Work out the finished part from the listing and answer in its coordinate system (mm). Face numbers are marked on the shaded views. Round coordinates to 2 decimals unless told otherwise and drop trailing zeros. Write each loop counter-clockwise with the first axis right and the second up, starting at its lowest first coordinate (ties: lowest second). Pieces come first, ordered by that corner, then holes. Notation, with made-up numbers: (12.25, 16.25) - (69.25, 16.25) arc R16 ccw to (69.25, 40.25) - close; hole circle Ø8 at (1.25, -20.5). An arc over 180 degrees is marked (long way). Answer as a JSON object with one key per item and string values.
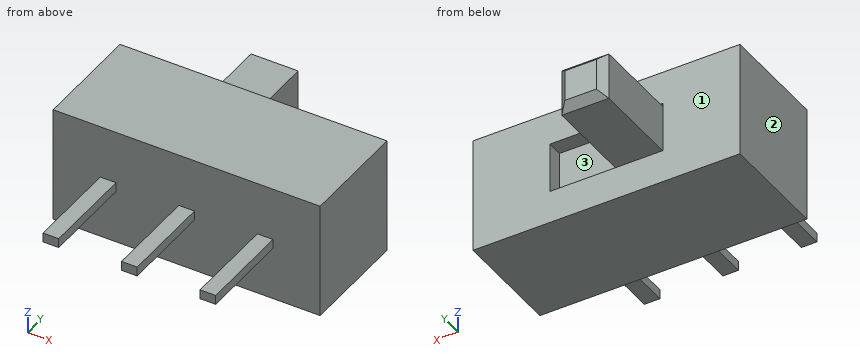
Autodesk Inventor part; units mm, degrees
ref_plane "YZ Plane" through (0, 0, 0) normal (1, 0, 0) x (0, 1, 0)
ref_plane "XZ Plane" through (0, 0, 0) normal (0, 1, 0) x (-1, 0, 0)
ref_plane "XY Plane" through (0, 0, 0) normal (0, 0, 1) x (1, 0, 0)
sketch "Sketch1" plane through (0, 0, 0) normal (0, 1, 0) x (-1, 0, 0)
  line L0 (4.25, -1.85) -> (-4.25, -1.85)
  line L1 (-4.25, -1.85) -> (-4.25, 1.85)
  line L2 (-4.25, 1.85) -> (4.25, 1.85)
  line L3 (4.25, 1.85) -> (4.25, -1.85)
  point P0 (0, 0)
  point P1 (4.25, 0)
  point P2 (0, -1.85)
  dimension "d0" = 8.5
  dimension "d1" = 3.7
extrude "Extrusion1" add sketch "Sketch1" along normal blind 3.5
sketch "Sketch2" plane through (0, 0, 0) normal (0, -1, 0) x (1, 0, 0)
  line L0 (4.25, 1.85) -> (-4.25, 1.85)
  line L1 (-2.75, 0.15) -> (-2.25, 0.15)
  line L2 (-2.25, 0.15) -> (-2.25, -0.15)
  line L3 (-2.25, -0.15) -> (-2.75, -0.15)
  line L4 (-2.75, -0.15) -> (-2.75, 0.15)
  line L5 (-0.25, 0.15) -> (0.25, 0.15)
  line L6 (0.25, 0.15) -> (0.25, -0.15)
  line L7 (0.25, -0.15) -> (-0.25, -0.15)
  line L8 (-0.25, -0.15) -> (-0.25, 0.15)
  line L9 (2.25, 0.15) -> (2.75, 0.15)
  line L10 (2.75, 0.15) -> (2.75, -0.15)
  line L11 (2.75, -0.15) -> (2.25, -0.15)
  line L12 (2.25, -0.15) -> (2.25, 0.15)
  point P0 (0, 0)
  point P1 (-2.75, 0)
  point P2 (-2.5, 0.15)
  point P3 (-0.25, 0)
  point P4 (0, 0.15)
  point P5 (2.25, 0)
  point P6 (2.5, 0.15)
  dimension "d4" = 0.5
  dimension "d5" = 0.3
  dimension "d6" = 2.5
  dimension "d9" = 2.5
extrude "Extrusion2" add sketch "Sketch2" along normal blind 3
sketch "Sketch3" plane through (0, 3.5, 0) normal (0, 1, 0) x (1, 0, 0)
  line L0 (-1.8, 0.8) -> (1.8, 0.8)
  line L1 (1.8, 0.8) -> (1.8, -0.8)
  line L2 (1.8, -0.8) -> (-1.8, -0.8)
  line L3 (-1.8, -0.8) -> (-1.8, 0.8)
  point P0 (0, 0)
  point P1 (-1.8, 0)
  point P2 (0, 0.8)
  dimension "d16" = 1.6
  dimension "d17" = 3.6
extrude "Extrusion3" cut sketch "Sketch3" against normal blind 0.5
sketch "Sketch4" plane through (0, 3, 0) normal (0, 1, 0) x (1, 0, 0)
  line L0 (-1.8, -0.8) -> (-1.8, 0.8)
  line L1 (-1.75, 0.75) -> (-0.25, 0.75)
  line L2 (-0.25, 0.75) -> (-0.25, -0.75)
  line L3 (-0.25, -0.75) -> (-1.75, -0.75)
  line L4 (-1.75, -0.75) -> (-1.75, 0.75)
  point P0 (0, 0)
  point P1 (-1.75, 0)
  dimension "d20" = 1.5
  dimension "d21" = 0.05
extrude "Extrusion4" add sketch "Sketch4" along normal blind 3.5
chamfer "Chamfer1" distance 0.25 angle 45 4 edges at (-1, 6.5, 0.75) (-0.25, 6.5, 0) (-1, 6.5, -0.75) (-1.75, 6.5, 0)
properties part number "Pololu #1408 Mini Slide Switch"
Item 1: A cutting plane is placed at C-C (x = 2.5). Write down the section's boundary in (y, z).
Results found:
{"outline": "(-3, -0.15) - (0, -0.15) - (0, -1.85) - (3.5, -1.85) - (3.5, 1.85) - (0, 1.85) - (0, 0.15) - (-3, 0.15) - close"}
Item 2: A cutting plane is placed at A-A (y = -0.75). Write down the section's boundary in (x, z), and give its area (3 significant figures).
Results found:
{"outline": "(-2.75, -0.15) - (-2.25, -0.15) - (-2.25, 0.15) - (-2.75, 0.15) - close; (-0.25, -0.15) - (0.25, -0.15) - (0.25, 0.15) - (-0.25, 0.15) - close; (2.25, -0.15) - (2.75, -0.15) - (2.75, 0.15) - (2.25, 0.15) - close", "area": "0.450 mm²"}
Item 3: Each of these flat-tipped pins is pushed along its axis until it touches: P1, Ø0.8, axis at x = -1.5, y = 5, coming from the -Z side; P2, Ø0.6, axis at x = 0, y = -1, coming from the -Z side; P3, Ø1.5, axis at y = -1.5, z = 0, coming from the -X side. Where does it stop, or does it pass through?
Results found:
{"P1": "z = -0.75", "P2": "z = -0.15", "P3": "x = -2.75"}
Item 4: A cutting plane is placed at D-D (y = 5.5). Write down the section's boundary in (x, z).
Results found:
{"outline": "(-1.75, -0.75) - (-0.25, -0.75) - (-0.25, 0.75) - (-1.75, 0.75) - close"}
Item 5: A cutting plane is placed at B-B (z = 0). Write down the section's boundary in (x, y).
Results found:
{"outline": "(-4.25, 0) - (-2.75, 0) - (-2.75, -3) - (-2.25, -3) - (-2.25, 0) - (-0.25, 0) - (-0.25, -3) - (0.25, -3) - (0.25, 0) - (2.25, 0) - (2.25, -3) - (2.75, -3) - (2.75, 0) - (4.25, 0) - (4.25, 3.5) - (1.8, 3.5) - (1.8, 3) - (-0.25, 3) - (-0.25, 6.25) - (-0.5, 6.5) - (-1.5, 6.5) - (-1.75, 6.25) - (-1.75, 3) - (-1.8, 3) - (-1.8, 3.5) - (-4.25, 3.5) - close"}
Item 6: Determine the mould class of the marked faces 1, 2 and 3 for opening direction X: pulls with the +X half, pulls with the -X half, needs draft (parallel to the pull), parting line crosses it, or undercut.
Results found:
{"face 1": "needs draft", "face 2": "pulls with the -X half", "face 3": "undercut"}
Item 7: Consider line 1 along Y through (x, z) = (-2.75, -0.6); line 2 along Y through (x, z) = (0, 0.4); line 3 along Z through (x, y) = (-0.75, 4.75). Determine where each line is inside the solid, lowest interval first.
Results found:
{"line 1": "0 to 3.5", "line 2": "0 to 3", "line 3": "-0.75 to 0.75"}
